Here's how the part is built. I have some questions about the finished solid (model axes, mm). Coordinates: 2 decimals unless noted, no trailing zeros. Loops run counter-clockwise (first coordinate to the right, second up) from the corner with the lowest first, then second, coordinate; pieces in that order, holes last. Notation, with made-up numbers: M 4.25,15.25 L 18.25,15.25 A27 cw 18.25,45.25 Z; hole C 1.5,13 d11. An arc over 180 degrees is marked long. Use CSV: the item, a comma, the result in double quotes. Start each with the question number.
Q1. If we section it at B-B (z = 14): Please give me the cut outline in (x, y), and give its area (3 significant figures).
Q2. If we section it at A-A (z = 1.5): Please give me the cut outline in (x, y).
Q3. Please list where these lines run through material, in increasing order: probe 1 along Y at (x, z) = (0, 7.5); probe 2 along Y at (x, z) = (0, 1.9); probe 3 along Z at (x, y) = (13, 1). Write a range as [from, to].
Q4. For pin 1 Ø2 at (x, z) = (9, 5) entering from +Y; pin 2 Ø3 at (x, z) = (-45, 7.5) entering from +Y; pin 3 Ø2 at (y, z) = (-3, 4.5) entering from -X; pin 4 Ø4 at (y, z) = (-1, 6) entering from +X, each with a flat end and sliding along its axis, tell me the tip position at first contact or that it passes through.
Q5. If we mould it in two halves opening along Y, with no side actions, what happens to faces 1 (the cylindrical face through (53.557, 16.866, 10.296)), 2 (the flat face through (17, 54, 18)), 3 (the cylindrical face through (-59.94, 2.64, 8.87)), 4 (the flat face through (-1, 1, 3))? For each: +Y half, -Y half, draft (parallel to the pull), parting line (faces both ways), or undercut.
from build123d import *

# Parameters (mm, degrees)
F0_R     = 60
F1_DEPTH = 3
F2_R     = 60
F2_R_2   = 56.15
F3_DEPTH = 15
F5_D     = 2
F6_R     = 0.2


with BuildPart() as f1:
    # F0 (on Top) → F1 (new body)
    with BuildSketch(Plane.XY):
        Circle(F0_R)
    extrude(amount=F1_DEPTH)

    # F2 (on face) → F3 (join)
    with BuildSketch(Plane.XY.offset(3)):
        Circle(F2_R)
        Circle(F2_R_2, mode=Mode.SUBTRACT)
    extrude(amount=F3_DEPTH)

    # F5 (through all)
    with Locations(Plane(origin=(0, 0, 0), x_dir=(1, 0, 0), z_dir=(0, 0, -1))):
        with Locations((0, 0)):
            Hole(F5_D / 2)

    # F6
    f6_edges = [f1.edges().sort_by_distance(p)[0] for p in [
        (-56.15, 0, 18),
    ]]
    fillet(f6_edges, radius=F6_R)


solid = f1.part
Results below:
1,outline,"C 0,0 d120; hole C 0,0 d112.3"
1,area,"1,400 mm^2"
2,outline,"C 0,0 d120; hole C 0,0 d2"
3,probe 1,"[-60, -56.15], [56.15, 60]"
3,probe 2,"[-60, -1], [1, 60]"
3,probe 3,"[0, 3]"
4,pin 1,"y = 59.46"
4,pin 2,"y = 41.32"
4,pin 3,"x = -59.97"
4,pin 4,"x = 60"
5,face 1,"undercut"
5,face 2,"draft"
5,face 3,"parting line"
5,face 4,"undercut"
